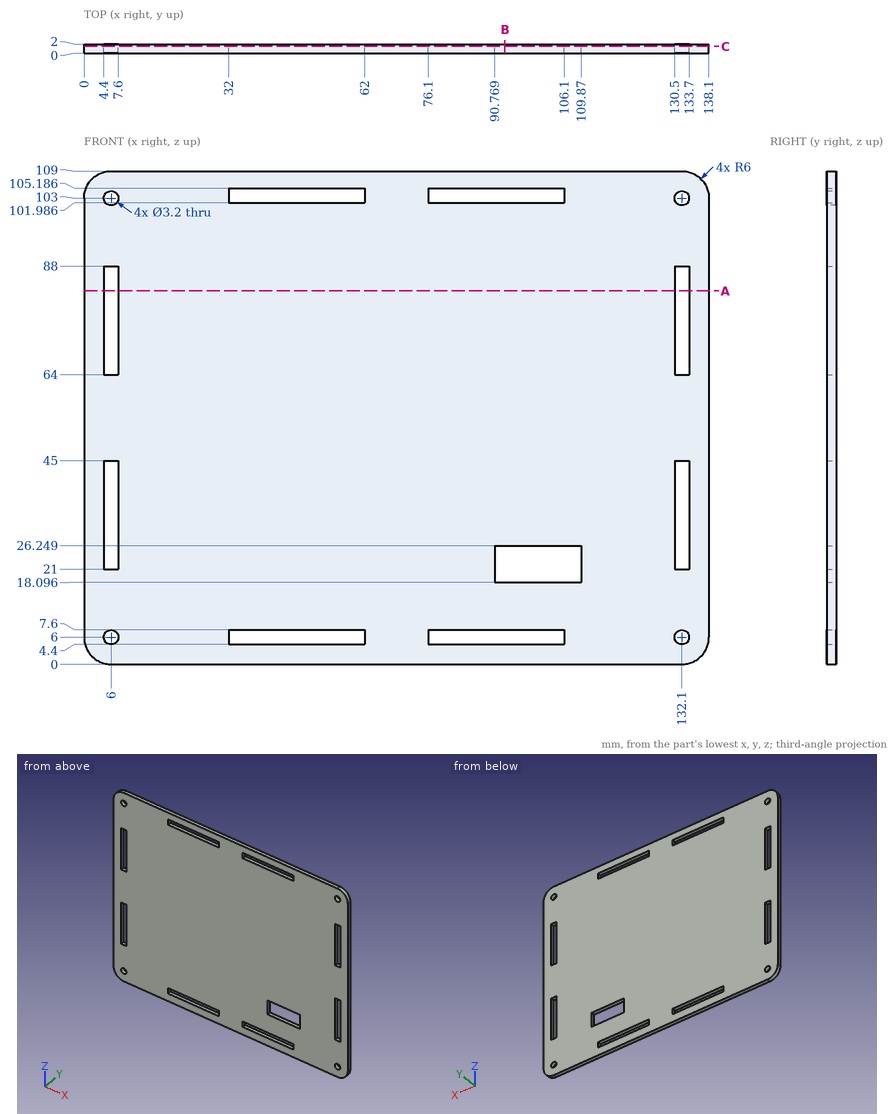
Check sheet for the drawn part. Datum: minimum x, y, z corner. Units: mm. Round coordinates to 2 decimals unless told otherwise and drop trailing zeros. Order: outer loops, then holes, each group sorted by start corner. A loop starts at its lowest first (then second) coordinate and runs counter-clockwise, first axis right, second up.
1) Section check B-B (x = 93). Record the boundary of the cut face in (y, z), and give its area (3 significant figures).
2) Scan lines: line 1 (X direction, y = 0.55, z = 77); line 2 (Z direction, x = 132.1, y = 0.4); line 3 (Z direction, x = 59, y = 1.7). Record each from-to range of solid material in increasing order.
3) Go/stop test with flat-tipped pins: pin 1 Ø0.6 at (y, z) = (1, 104) entering from -X; pin 2 Ø0.6 at (x, y) = (5, 1.5) entering from -Z; pin 3 Ø2.5 at (x, z) = (132.1, 6) entering from +Y. Record where each tip stops, or that it passes through.
4) Section check A-A (z = 82.5). Record the boundary of the cut face in (x, y), and give its area (3 significant figures).
5) Section check C-C (y = 1.5). Give the number of separate pieces and of enclosed holes in the cut face, and give its area (3 significant figures).
Result:
1. outline: (0, 0) - (2, 0) - (2, 4.4) - (0, 4.4) - close; (0, 7.6) - (2, 7.6) - (2, 18.1) - (0, 18.1) - close; (0, 26.25) - (2, 26.25) - (2, 101.99) - (0, 101.99) - close; (0, 105.19) - (2, 105.19) - (2, 109) - (0, 109) - close
1. area: 189 mm2
2. line 1: x = 0 to 4.4, 7.6 to 130.5, 133.7 to 138.1
2. line 2: z = 0 to 4.4, 7.6 to 21, 45 to 64, 88 to 101.4, 104.6 to 109
2. line 3: z = 0 to 4.4, 7.6 to 101.99, 105.19 to 109
3. pin 1: stops at x = 0.04
3. pin 2: stops at z = 0.04
3. pin 3: passes through
4. outline: (0, 0) - (4.4, 0) - (4.4, 2) - (0, 2) - close; (7.6, 0) - (130.5, 0) - (130.5, 2) - (7.6, 2) - close; (133.7, 0) - (138.1, 0) - (138.1, 2) - (133.7, 2) - close
4. area: 263 mm2
5. separate pieces: 1
5. enclosed holes: 13
5. area: 14,100 mm2
